Model file for the job. Use its own axes, mm. Face numbers are marked on the shaded views. A direction names the side the tool comes from. Round coordinates to 2 decimals unless told otherwise and drop trailing zeros. Loops run counter-clockwise (first coordinate to the right, second up) from the corner with the lowest first, then second, coordinate; pieces in that order, holes last. Notation, with made-up numbers: (62.25, 51.5) - (72.25, 51.5) arc R19 cw to (72.25, 77.5) - close; hole circle Ø7 at (60, 37). An arc over 180 degrees is marked (long way). Use one line per item in the form item = value.
Autodesk Inventor part; units mm, degrees
ref_plane "YZ Plane" through (0, 0, 0) normal (1, 0, 0) x (0, 1, 0)
ref_plane "XZ Plane" through (0, 0, 0) normal (0, 1, 0) x (-1, 0, 0)
ref_plane "XY Plane" through (0, 0, 0) normal (0, 0, 1) x (1, 0, 0)
sketch "スケッチ1" plane through (0, 0, 0) normal (1, 0, 0) x (0, 1, 0)
  circle A0 centre (0, 0) radius 5.1
  line L0 (1, 15) -> (6, 15)
  line L1 (6, 15) -> (6, -15)
  line L2 (6, -15) -> (1, -15)
  line L3 (1, -15) -> (1, 15)
  circle A1 centre (0, 0) radius 8.1
  point P0 (1, 5.001)
  point P1 (1, -5.001)
  point P2 (6, -5.4415)
  point P3 (6, 5.4415)
  dimension "d0" = 10.2
  dimension "d1" = 1
  dimension "d2" = 30
  dimension "d3" = 15
  dimension "d4" = 5
  dimension "d5" = 3
extrude "押し出し1" add sketch "スケッチ1" against normal blind 10 contours A0 L3 A1 L1 | L3 L0 L1 A1 | A1 L1 L2 L3 | A1 L1
sketch "スケッチ2" plane through (0, 6, 15) normal (0, 1, 0) x (1, 0, 0)
  line L0 (0, 9.5585) -> (0, 0)
  line L1 (0, 0) -> (-10, 0)
  line L2 (0, 30) -> (0, 20.4415)
  line L3 (0, 30) -> (-10, 30)
  point P0 (0, 15)
  point P1 (-5, 5)
  point P2 (-5, 25)
  dimension "d8" = 5
  dimension "d9" = 5
  dimension "d10" = 5
  dimension "d11" = 5
hole "穴1" at (-5, 6, 10) at (-5, 6, -10) direction (0, -1, 0) diameter 3.2 end through all
fillet "フィレット1" radius 2 6 edges at (0, 3.5, 15) (-10, 3.5, 15) (-5, 6, 5.4415) (-5, 6, -5.4415) (0, 3.5, -15) (-10, 3.5, -15)
properties part number "belt_liner_v5_3DP_P-2" material "ABS プラスチック"
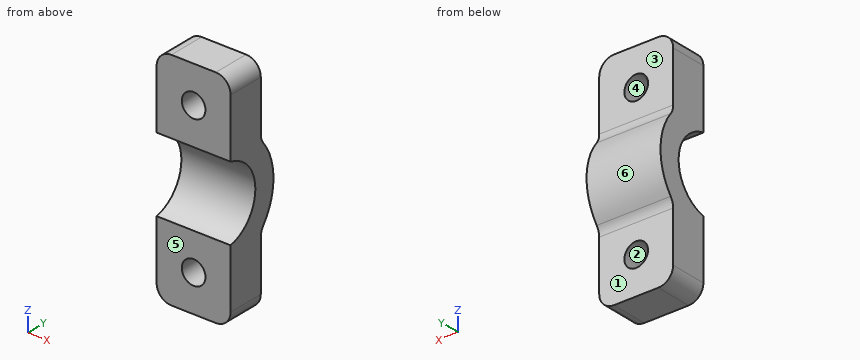
1. Flat gauge pins, fed straight in: pin 1 (2.5 mm diameter, centred on x = -3.5, z = -9.5, fed in from +Y); pin 2 (6 mm diameter, centred on x = -7.5, z = -8, fed in from +Y); pin 3 (6 mm diameter, centred on x = -1.5, z = 1, fed in from -Y). Where does each tip first touch, or does it go through?
Geometry check:
pin_1 = 6
pin_2 = 6.37
pin_3 = 3.16
2. Tool access for the marked faces 1, 2 and 3: list every direction of +Z, -Z, +X, -X, +Y, -Y with a clear straight run to the whole face (end or side of a thin tool).
Geometry check:
face_1 = -Z, +X, -X, +Y
face_2 = +Y, -Y
face_3 = +Z, +X, -X, +Y
3. Cut at C-C, the plane x = -5. Give the cut face in (y, z), plus the area to 3 significant figures.
Geometry check:
outline = (1, -15) - (6, -15) - (6, -11.6) - (1, -11.6) - close; (1, -8.4) - (6, -8.4) - (6, -6.17) arc R2 cw to (6.42, -4.94) arc R8.1 ccw to (6.42, 4.94) arc R2 cw to (6, 6.17) - (6, 8.4) - (1, 8.4) - (1, 5) arc R5.1 cw to (1, -5) - close; (1, 11.6) - (6, 11.6) - (6, 15) - (1, 15) - close
area = 103 mm^2
4. Cut at D-D, the plane x = -6.25. Give the cut face in (y, z), plus the area to 3 significant figures.
Geometry check:
outline = (1, -15) - (6, -15) - (6, -11) - (1, -11) - close; (1, -9) - (6, -9) - (6, -6.17) arc R2 cw to (6.42, -4.94) arc R8.1 ccw to (6.42, 4.94) arc R2 cw to (6, 6.17) - (6, 9) - (1, 9) - (1, 5) arc R5.1 cw to (1, -5) - close; (1, 11) - (6, 11) - (6, 15) - (1, 15) - close
area = 115 mm^2
5. Wall check: probe 1 along X at (y, z) = (2.3, -10); probe 2 along Z at (x, y) = (-4, 3.5); probe 3 along Z at (x, y) = (-5, 2.75). Give the ranges that are in metal, low to high.
Geometry check:
probe_1 = -10 to -6.6, -3.4 to 0
probe_2 = -15 to -11.25, -8.75 to -3.71, 3.71 to 8.75, 11.25 to 15
probe_3 = -15 to -11.6, -8.4 to -4.3, 4.3 to 8.4, 11.6 to 15
6. Cut at A-A, the plane z = -10. Give the cut face in (x, y), plus the area to 3 significant figures.
Geometry check:
outline = (-10, 1) - (-6.6, 1) - (-6.6, 6) - (-10, 6) - close; (-3.4, 1) - (0, 1) - (0, 6) - (-3.4, 6) - close
area = 34.0 mm^2
7. Pull direction Z, two halves, no side cores. Call the marked faces 4, 5 and 6: +Z half, -Z half, draft (parallel to the pull), parting line (faces both ways), or undercut.
Geometry check:
face_4 = undercut
face_5 = draft
face_6 = parting line
8. Cut at B-B, the plane y = 3.75. Give the cut face in (x, z).
Geometry check:
outline = (-10, -13) arc R2 ccw to (-8, -15) - (-2, -15) arc R2 ccw to (0, -13) - (0, -3.46) - (-10, -3.46) - close; (-10, 3.46) - (0, 3.46) - (0, 13) arc R2 ccw to (-2, 15) - (-8, 15) arc R2 ccw to (-10, 13) - close; hole circle Ø3.2 at (-5, -10); hole circle Ø3.2 at (-5, 10)
